For this review, take the finished solid that the model builds, in its own axes (mm). Face numbers are marked on the shaded views. A direction names the side the tool comes from. Coordinates: 2 decimals unless noted, no trailing zeros. Write each loop counter-clockwise with the first axis right and the second up, starting at its lowest first coordinate (ties: lowest second). Pieces come first, ordered by that corner, then holes. Notation, with made-up numbers: (66.25, 69.5) -> (121.25, 69.5) arc R17 cw to (121.25, 81.5) -> close; hole circle Ø9 at (40, 35.5). An arc over 180 degrees is marked (long way). Put each result on its own line as item: value. Start each with the question number.
Item 1: Consider section B-B on x = -6.5. Give the boundary of the cut face in (y, z), and give its area (3 significant figures).
Item 2: Consider section A-A on y = 10.5. Give the number of separate pieces and of enclosed holes in the cut face, and give its area (3 significant figures).
Item 3: Consider section C-C on x = -31.75. Give the boundary of the cut face in (y, z).
Item 4: To check wall thickness, follow L1, parallel to Y at x = -24.5, z = -59.8; L2, parallel to Z at x = -8.5, y = 4; L3, parallel to X at y = 10, z = -1. State the ranges of each line that lie inside material, in increasing order.
Item 5: For the marked faces 1, 2 and 3, list the 3-axis set-ups (+Z, -Z, +X, -X, +Y, -Y) from which the entire face can be reached by the end or side of a thin tool; tool diameter is ignored.
Item 6: Insertion check: P1, Ø15, axis at x = -9, z = -51, coming from the +Y side; P2, Ø1.3, axis at x = -24.5, y = 17.75, coming from the -Z side; P3, Ø6, axis at x = -20.5, z = -6.5, coming from the -Y side; P4, Ø5, axis at y = 16, z = -25.5, coming from the -X side. Each pin has a flat end and moves straight along its axis. Give the tip position at first contact, or say it passes through.
Autodesk Inventor part; units mm, degrees
ref_plane "YZ Plane" through (0, 0, 0) normal (1, 0, 0) x (0, 1, 0)
ref_plane "XZ Plane" through (0, 0, 0) normal (0, 1, 0) x (-1, 0, 0)
ref_plane "XY Plane" through (0, 0, 0) normal (0, 0, 1) x (1, 0, 0)
sketch "Sketch1" plane through (0, 0, 0) normal (0, 1, 0) x (-1, 0, 0)
  line L0 (0, 0) -> (0, -58)
  line L1 (0, -58) -> (35, -58)
  line L2 (35, -58) -> (35, -62)
  line L3 (35, -62) -> (-4, -62)
  line L4 (-4, -62) -> (-4, 0)
  line L5 (-4, 0) -> (0, 0)
  line L6 (0, 0) -> (35, 0)
  line L7 (35, 0) -> (35, -4)
  line L8 (35, -4) -> (0, -4)
  line L9 (0, -4) -> (0, 0)
  dimension "d0" = 58
  dimension "d1" = 35
  dimension "d2" = 4
  dimension "d3" = 39
  dimension "d27" = 35
  dimension "d28" = 4
extrude "Extrusion1" add sketch "Sketch1" along normal blind 21
sketch "Sketch2" plane through (4, 0, 0) normal (1, 0, 0) x (0, 0, -1)
  line L0 (0, 21) -> (62, 21)
  line L1 (0, 21) -> (25.5, 21)
  line L2 (25.5, 21) -> (25.5, 16)
  line L3 (25.5, 16) -> (0, 16)
  line L4 (0, 16) -> (0, 21)
  line L5 (25.5, 16) -> (36.5, 16)
  line L6 (36.5, 16) -> (36.5, 5)
  line L7 (36.5, 5) -> (25.5, 5)
  line L8 (25.5, 5) -> (25.5, 16)
  circle A0 centre (25.5, 16) radius 1.5
  circle A1 centre (36.5, 16) radius 1.5
  circle A2 centre (25.5, 5) radius 1.5
  circle A3 centre (36.5, 5) radius 1.5
  point P0 (0, 0)
  dimension "d6" = 25.5
  dimension "d7" = 5
  dimension "d8" = 11
  dimension "d9" = 11
  dimension "d10" = 3
  dimension "d11" = 3
  dimension "d12" = 3
  dimension "d13" = 3
extrude "Extrusion2" cut sketch "Sketch2" against normal blind 21 contours A0 L5 L2 | L2 L3 A0 | L3 L8 A0 | L5 A0 L8 | A1 L6 L5 | L5 L6 A1 | A2 L7 L8 | L8 L7 A2 | A3 L7 L6 | L6 L7 A3
sketch "Sketch3" plane through (-35, 0, -58) normal (0, 0, 1) x (1, 0, 0)
  line L0 (0, 0) -> (0, 21)
  line L1 (0, 10.5) -> (10.5, 10.5)
  circle A0 centre (10.5, 10.5) radius 10.5
  line L2 (0, 21) -> (10.5, 21)
  line L3 (10.5, 21) -> (10.5, 0)
  line L4 (10.5, 0) -> (0, 0)
  line L5 (0, 0) -> (0, 21)
  circle A1 centre (10.5, 10.5) radius 8
  circle A2 centre (10.5, 10.5) radius 6.5
  line L6 (10.5, 18.5) -> (10.5, 17)
  line L7 (10.5, 4) -> (10.5, 2.5)
  line L8 (2.5, 10.5) -> (4, 10.5)
  line L9 (10.5, 10.5) -> (18.5, 10.5)
  line L10 (18.5, 10.5) -> (17, 10.5)
  circle A3 centre (10.5, 17.75) radius 1.1
  circle A4 centre (3.25, 10.5) radius 1.1
  circle A5 centre (17.75, 10.5) radius 1.1
  circle A6 centre (10.5, 3.25) radius 1.1
  circle A7 centre (10.5, 10.5) radius 3
  point P0 (35, 0)
  point P1 (10.5, 21)
  dimension "d16" = 10.5
  dimension "d17" = 16
  dimension "d18" = 13
  dimension "d19" = 2.2
  dimension "d20" = 2.2
  dimension "d21" = 2.2
  dimension "d22" = 2.2
  dimension "d23" = 6
extrude "Extrusion3" cut sketch "Sketch3" along normal mid plane 1000 contours L0 A0 L4 | L0 L2 A0 | A4 A1 L1 | L1 A1 A4 | A6 A1 L3 | L3 A1 A6 | A1 A4 A2 L1 | L1 A2 A4 A1 | A3 A1 L3 | L3 A1 A3 | A1 A6 A2 L3 | L3 A2 A6 A1 | A2 A4 L1 | L1 A4 A2 | A1 L3 A2 A3 | A1 A3 A2 L3 | A2 A6 L3 | L3 A6 A2 | A5 A2 L9 A1 | A1 A5 | A2 L3 A3 | A2 A3 L3 | A1 L9 A2 A5 | A5 L9 A2 | A7 L3 L1 | L1 L3 A7 | A2 L9 A5 | L3 L9 A7 | L3 A7 L9
fillet "Fillet1" radius 4 2 edges at (0, 10.5, -58) (0, 10.5, -4)
sketch "Sketch4" plane through (4, 0, 0) normal (1, 0, 0) x (0, 0, -1)
  circle A0 centre (25.5, 16) radius 1.5
  line L0 (25.5, 16) -> (20.5, 16)
  line L1 (20.5, 16) -> (41.5, 16)
  line L2 (20.5, 16) -> (41.5, 16)
  line L3 (41.5, 16) -> (41.5, 31)
  line L4 (41.5, 31) -> (20.5, 31)
  line L5 (20.5, 31) -> (20.5, 16)
  circle A1 centre (25.5, 5) radius 1.5
  line L6 (25.5, 5) -> (20.5, 5)
  circle A2 centre (36.5, 5) radius 1.5
  line L7 (20.5, 5) -> (36.5, 5)
  line L8 (36.5, 5) -> (41.5, 5)
  line L9 (20.5, 5) -> (41.5, 5)
  line L10 (41.5, 5) -> (41.5, -10)
  line L11 (41.5, -10) -> (20.5, -10)
  line L12 (20.5, -10) -> (20.5, 5)
  line L13 (0, 21) -> (62, 21)
  line L14 (20.5, 31) -> (41.5, 31)
  line L15 (41.5, 31) -> (41.5, 21)
  line L16 (41.5, 21) -> (20.5, 21)
  line L17 (20.5, 21) -> (20.5, 31)
  line L18 (41.5, -10) -> (20.5, -10)
  line L19 (20.5, -10) -> (20.5, -2.5)
  line L20 (41.5, -2.5) -> (41.5, -10)
  line L21 (20.5, -10) -> (41.5, -10)
  line L22 (41.5, -10) -> (41.5, 0)
  line L23 (41.5, 0) -> (20.5, 0)
  line L24 (20.5, 0) -> (20.5, -10)
  line L25 (20.5, 31) -> (41.5, 31)
  line L26 (41.5, 31) -> (41.5, 21)
  line L27 (41.5, 21) -> (20.5, 21)
  line L28 (20.5, 21) -> (20.5, 31)
  point P0 (0, 0)
  point P1 (38, 5)
  point P2 (35, 5)
  point P3 (27, 5)
  point P4 (24, 5)
  dimension "d29" = 5
  dimension "d30" = 21
  dimension "d31" = 15
  dimension "d32" = 15
extrude "Extrusion4" add sketch "Sketch4" against normal blind 4 contours L13 L5 L4 L3 | L7 A2 L8 L10 L23 L12 L6 A1 | L23 L10 L11 L12
fillet "Fillet2" radius 2 4 edges at (2, 21, -41.5) (2, 21, -20.5) (2, 0, -41.5) (2, 0, -20.5)
fillet "Fillet3" radius 11 4 edges at (2, 31, -20.5) (2, 31, -41.5) (2, -10, -20.5) (2, -10, -41.5)
properties part number "L2"
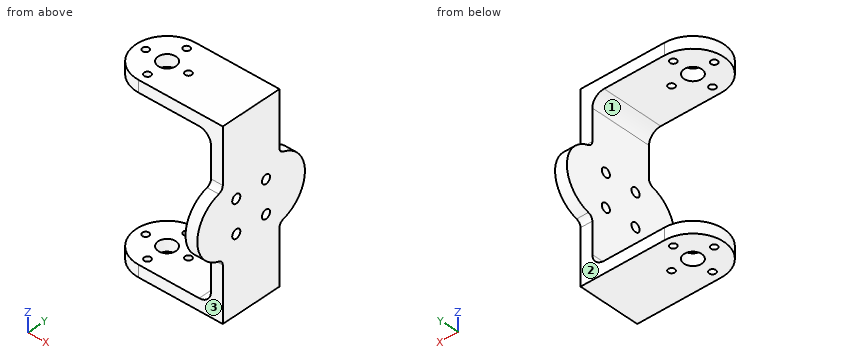
Return value:
1. outline: (0, -62) -> (21, -62) -> (21, -58) -> (0, -58) -> close; (0, -4) -> (21, -4) -> (21, 0) -> (0, 0) -> close
1. area: 168 mm^2
2. separate pieces: 7
2. enclosed holes: 0
2. area: 452 mm^2
3. outline: (2.9, -62) -> (9.4, -62) -> (9.4, -58) -> (2.9, -58) -> close; (2.9, -4) -> (9.4, -4) -> (9.4, 0) -> (2.9, 0) -> close; (11.6, -62) -> (18.1, -62) -> (18.1, -58) -> (11.6, -58) -> close; (11.6, -4) -> (18.1, -4) -> (18.1, 0) -> (11.6, 0) -> close
4. L1: 0 to 2.15, 4.35 to 7.5, 13.5 to 16.65, 18.85 to 21
4. L2: -62 to -58, -4 to 0
4. L3: -34.99 to -32.73, -30.77 to -27.46, -21.54 to -18.23, -16.27 to 4
5. face 1: -X, +Y, -Y
5. face 2: -Z, +X, -X, +Y
5. face 3: -Z, +X, -X, -Y
6. P1: y = 21
6. P2: through
6. P3: y = 0
6. P4: x = 0
